```python
from build123d import *

# Parameters (mm, degrees)
SKETCH_4_W            = 47.1
SKETCH_4_H            = 29.6
EXTRUDE_256_DEPTH     = 37.9
SKETCH_8_W            = 47.1
SKETCH_8_H            = 32
CUT_EXTRUDE_1_DEPTH   = 2.2
SKETCH_12_W           = 47.1
SKETCH_12_H           = 2.9
CUT_EXTRUDE_619_DEPTH = 26.6
CUT_EXTRUDE_3_DEPTH   = 3
SKETCH_17_R           = 3
EXTRUDE_1677_DEPTH    = 10.3
SKETCH_19_R           = 12.2
EXTRUDE_1895_DEPTH    = 30.8


with BuildPart() as part:
    # 草图4 → Extrude 256 (new body)
    with BuildSketch(Plane.XY):
        Rectangle(SKETCH_4_W, SKETCH_4_H)
    extrude(amount=EXTRUDE_256_DEPTH)

    # 草图8 → 切除-拉伸1 (cut)
    with BuildSketch(Plane.XZ.offset(14.8)):
        with Locations((0, 16)):
            Rectangle(SKETCH_8_W, SKETCH_8_H)
    extrude(amount=-CUT_EXTRUDE_1_DEPTH, mode=Mode.SUBTRACT)

    # 草图12 → Cut-Extrude 619 (cut)
    with BuildSketch(Plane.XZ.offset(14.8)):
        with Locations((0, 33.45)):
            Rectangle(SKETCH_12_W, SKETCH_12_H)
    extrude(amount=-CUT_EXTRUDE_619_DEPTH, mode=Mode.SUBTRACT)

    # 草图14 → 切除-拉伸3 (cut)
    with BuildSketch(Plane.XY.offset(37.9)):
        with BuildLine():
            ThreePointArc((-14.55, 5.9), (-15.106497116, 7.243502884), (-16.45, 7.8))
            Line((-16.45, 7.8), (-16.65, 7.8))
            ThreePointArc((-16.65, 7.8), (-17.993502884, 7.243502884), (-18.55, 5.9))
            Line((-18.55, 5.9), (-18.55, -7.9))
            ThreePointArc((-18.55, -7.9), (-17.993502884, -9.243502884), (-16.65, -9.8))
            Line((-16.65, -9.8), (-16.45, -9.8))
            ThreePointArc((-16.45, -9.8), (-15.106497116, -9.243502884), (-14.55, -7.9))
            Line((-14.55, -7.9), (-14.55, 5.9))
        make_face()
    cut_extrude_3 = extrude(amount=-CUT_EXTRUDE_3_DEPTH, mode=Mode.SUBTRACT)

    # 镜向3: 切除-拉伸3 across plane
    add(cut_extrude_3.mirror(Plane(origin=(0, 0, 0), x_dir=(0, 0, 1), z_dir=(1, 0, 0))), mode=Mode.SUBTRACT)

    # 草图17 → Extrude 1677 (add)
    with BuildSketch(Plane(origin=(0, 14.8, 0), x_dir=(1, 0, 0), z_dir=(0, 1, 0))):
        with Locations(Location((-7.95, -15.8, 0), (0, 0, 90))):
            Circle(SKETCH_17_R)
    extrude(amount=EXTRUDE_1677_DEPTH)

    # 草图19 → Extrude 1895 (add)
    with BuildSketch(Plane(origin=(23.55, 0, 0), x_dir=(0, 0, -1), z_dir=(1, 0, 0))):
        with Locations(Location((-13.6, -2.9, 0), (0, 0, 232.66299834))):
            Circle(SKETCH_19_R)
    extrude(amount=EXTRUDE_1895_DEPTH)


solid = part.part
```
Here's how the part is built. I have some questions about the finished solid (model axes, mm). A direction names the side the tool comes from. Round coordinates to 2 decimals unless told otherwise and drop trailing zeros. Loops run counter-clockwise (first coordinate to the right, second up) from the corner with the lowest first, then second, coordinate; pieces in that order, holes last. Notation, with made-up numbers: (27, 74.25) -> (40, 74.25) arc R13 cw to (40, 79.25) -> close; hole circle Ø8 at (-7.75, 29.25). An arc over 180 degrees is marked (long way). Answer as CSV lines item,"result". Start each with the question number.
1. Imagine slicing it at D-D on y = 16. Write out the boundary of the cut face in (x, z).
2. Imagine slicing it at C-C on z = 15.8. Write out the boundary of the cut face in (x, y), plus the area to 3 significant figures.
3. For faces 5 (the face through (38.734, 6.465, 5.781)), 6 (the face through (15.121, -9.258, 36.421)), 7 (the face through (0, -12.6, 16)), which set-ups out of +Z, -Z, +X, -X, +Y, -Y let a thin tool reach every point of the face, with its end or its side?
4. If we mould it in two halves opening along Y, with no side actions, what happens to faces 1 (the face through (-8, 25.1, 16)), 2 (the face through (-15.092, 7.229, 36.421)), 3 (the face through (-17.979, 7.258, 36.421)), 4 (the face through (23.55, -14, 14))? For each: pulls with the +Y half, pulls with the -Y half, needs draft (parallel to the pull), parting line crosses it, or undercut.
5. I need wall thicknesses on probe 1 along Z at (x, y) = (2.5, -5.5); probe 2 along Y at (x, z) = (-16, 5); probe 3 along X at (y, z) = (10, 13). Which ranges of each line are inside material? Lowest first, please. Write a range as from..to.
6. Imagine slicing it at A-A on y = -2.9. Write out the boundary of the cut face in (x, z), plus the area to 3 significant figures.
7. I'm going to push flat-ended pins straight in: P1, Ø3, axis at x = -15.5, z = 19, coming from the +Y side; P2, Ø5, axis at x = 18, z = 33, coming from the -Y side; P3, Ø9.5, axis at x = 6, z = 20.5, coming from the -Y side. Where does each tip first touch, or does it pass through?
8. Imagine slicing it at B-B on x = -7.95. Write out the boundary of the cut face in (y, z).
Solution:
1,outline,"circle Ø6 at (-7.95, 15.8)"
2,outline,"(-23.55, -12.6) -> (23.55, -12.6) -> (23.55, -14.9) -> (54.35, -14.9) -> (54.35, 9.1) -> (23.55, 9.1) -> (23.55, 14.8) -> (-4.95, 14.8) -> (-4.95, 25.1) -> (-10.95, 25.1) -> (-10.95, 14.8) -> (-23.55, 14.8) -> close"
2,area,"2,090 mm²"
3,face 5,"+X"
3,face 6,"+Z"
3,face 7,"-Z, -X, -Y"
4,face 1,"pulls with the +Y half"
4,face 2,"undercut"
4,face 3,"undercut"
4,face 4,"needs draft"
5,probe 1,"0..32, 34.9..37.9"
5,probe 2,"-12.6..14.8"
5,probe 3,"-23.55..23.55"
6,outline,"(-23.55, 0) -> (23.55, 0) -> (23.55, 1.4) -> (54.35, 1.4) -> (54.35, 25.8) -> (23.55, 25.8) -> (23.55, 32) -> (-23.55, 32) -> close; (-23.55, 34.9) -> (-18.55, 34.9) -> (-18.55, 37.9) -> (-23.55, 37.9) -> close; (-14.55, 34.9) -> (14.55, 34.9) -> (14.55, 37.9) -> (-14.55, 37.9) -> close; (18.55, 34.9) -> (23.55, 34.9) -> (23.55, 37.9) -> (18.55, 37.9) -> close"
6,area,"2,380 mm²"
7,P1,"y = 14.8"
7,P2,"y = -14.8"
7,P3,"y = -12.6"
8,outline,"(-14.8, 34.9) -> (11.8, 34.9) -> (11.8, 32) -> (-12.6, 32) -> (-12.6, 0) -> (14.8, 0) -> (14.8, 12.8) -> (25.1, 12.8) -> (25.1, 18.8) -> (14.8, 18.8) -> (14.8, 37.9) -> (-14.8, 37.9) -> close"
